Work out the finished part from the listing and answer in its coordinate system (mm). Face numbers are marked on the shaded views. Coordinates: 2 decimals unless noted, no trailing zeros. Write each loop counter-clockwise with the first axis right and the second up, starting at its lowest first coordinate (ties: lowest second). Pieces come first, ordered by that corner, then holes. Notation, with made-up numbers: (88.5, 33.25) - (129.5, 33.25) arc R23 ccw to (129.5, 50.25) - close; hole circle Ø7 at (61, 1.25). An arc over 180 degrees is marked (long way). Answer as a JSON object with one key per item and string values. Group by question number.
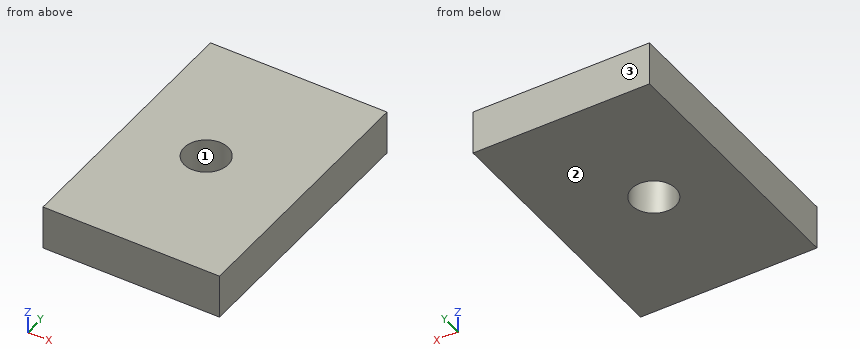
from build123d import *

# Parameters (mm, degrees)
SKETCH1_W               = 20
SKETCH1_H               = 30
BOSS_EXTRUDE1_DEPTH     = 5
CUT_EXTRUDE1_DEPTH      = 12
CUT_EXTRUDE1_DEPTH_BACK = 9
SKETCH2_R               = 2.5


with BuildPart() as part:
    # Sketch1 → Boss-Extrude1 (new body)
    with BuildSketch(Plane.XY):
        Rectangle(SKETCH1_W, SKETCH1_H)
    extrude(amount=BOSS_EXTRUDE1_DEPTH)

    # Sketch2 → Cut-Extrude1 (cut, two sides: drawn at the far end of the back side and taken through both)
    with BuildSketch(Plane.XY.offset(5).offset(-CUT_EXTRUDE1_DEPTH_BACK)):
        with Locations(Location((-1, 0, 0), (0, 0, 180))):
            Circle(SKETCH2_R)
    extrude(amount=CUT_EXTRUDE1_DEPTH + CUT_EXTRUDE1_DEPTH_BACK, mode=Mode.SUBTRACT)


solid = part.part
Q1. For a pull along Y with two mould halves and no side action, classify the marked faces 1, 2 and 3 as +Y half, -Y half, draft (parallel to the pull), parting line (faces both ways), or undercut.
Q2. Section B-B on x = -1 is taken. Determine the outline of the cut face in (y, z), plus the area to 3 significant figures.
Q3. Section A-A on y = 0 is taken. Determine the outline of the cut face in (x, z).
Q4. Consider L1, parallel to Y at x = -1, z = 3.75; L2, parallel to Y at x = 0.5, z = 3.75. Determine where each line is inside the solid, lowest interval first. Write a range as from..to.
Q5. Section C-C on z = 0.45 is taken. Determine the outline of the cut face in (x, y).
Q6. A flat-ended cylindrical pin translates along its axis: pin 1 Ø6 at (x, y) = (-1, 0) entering from +Z. Find the tip coordinate at first contact, or state that the pin passes through.
Numbers:
{
 "1": {"face 1": "undercut", "face 2": "draft", "face 3": "+Y half"},
 "2": {"outline": "(-15, 0) - (-2.5, 0) - (-2.5, 5) - (-15, 5) - close; (2.5, 0) - (15, 0) - (15, 5) - (2.5, 5) - close", "area": "125 mm²"},
 "3": {"outline": "(-10, 0) - (-3.5, 0) - (-3.5, 5) - (-10, 5) - close; (1.5, 0) - (10, 0) - (10, 5) - (1.5, 5) - close"},
 "4": {"L1": "y = -15..-2.5, 2.5..15", "L2": "y = -15..-2, 2..15"},
 "5": {"outline": "(-10, -15) - (10, -15) - (10, 15) - (-10, 15) - close; hole circle Ø5 at (-1, 0)"},
 "6": {"pin 1": "stops at z = 5"}
}
